Read the model definition and answer for the solid it produces. Units are mm, in the model's axes. A direction names the side the tool comes from. Coordinates: 2 decimals unless noted, no trailing zeros. Loops run counter-clockwise (first coordinate to the right, second up) from the corner with the lowest first, then second, coordinate; pieces in that order, holes last.
from build123d import *

# Parameters (mm, degrees)
F1_DEPTH = 30
F3_D     = 7
F5_D     = 7
F6_W     = 20.071618259
F6_H     = 16.8062914163
F7_DEPTH = 87


with BuildPart() as f1:
    # F0 (on Front) → F1 (new body)
    with BuildSketch(Plane.XZ):
        with BuildLine():
            ThreePointArc((-5.9981474183, 6.1490890598), (-4.2950281931, 1.8104018307), (0, 0))
            Line((0, 0), (40, 0))
            ThreePointArc((40, 0), (44.8583417204, 2.4791313959), (45.7018609438, 7.8678280909))
            Line((45.7018609438, 7.8678280909), (30, 100))
            Line((30, 100), (20, 100))
            Line((20, 100), (10, 100))
            Line((10, 100), (-5.9981474183, 6.1490890598))
        make_face()
        with BuildLine():
            ThreePointArc((30, 100), (20, 111.6119907276), (10, 100))
            Line((10, 100), (20, 100))
            Line((20, 100), (30, 100))
        make_face()
    extrude(amount=F1_DEPTH)

    # F3 (through all)
    with Locations(Plane.XZ.offset(30)):
        with Locations((20, 7.6905470341)):
            Hole(F3_D / 2)

    # F5 (through all)
    with Locations(Plane.XZ.offset(30)):
        with Locations((20, 101.5001014674)):
            Hole(F5_D / 2)

    # F6 (on face) → F7 (cut)
    with BuildSketch(Plane(origin=(0, 0, 0), x_dir=(1, 0, 0), z_dir=(0, 0, -1))):
        with Locations((20.9973212332, 14.0443919227)):
            Rectangle(F6_W, F6_H)
    extrude(amount=-F7_DEPTH, mode=Mode.SUBTRACT)


solid = f1.part
Q1. Which of the six approach directions +Z, -Z, +X, -X, +Y, -Y give full straight-line access (tool end or side, diameter ignored) to faces 5 (the face through (16.66, -26.17, 8.74)), 6 (the face through (21, -22.448, 43))?
Findings below:
face 5: +Y, -Y
face 6: -Z
Q2. A cutting plane is placed at C-C (y = -4.25). Give the vertices of the cut face in (x, z), then the cut area to 3 significant figures.
Findings below:
outline: (-6, 6.15) arc R6 ccw to (0, 0) - (40, 0) arc R6 ccw to (45.7, 7.87) - (30, 100) arc R10.11 ccw (long way) to (10, 100) - close; hole circle Ø7 at (20, 7.69); hole circle Ø7 at (20, 101.5)
area: 3,800 mm2
Q3. Determine the mould class of faces 1 (the face through (10.962, -14, 43)), 2 (the face through (20, 0, 44)), 3 (the face through (-4.342, -14.79, 1.859)), 4 (the face through (37.96, -14.79, 53.29)) for opening direction X: +X half, -X half, draft (parallel to the pull), parting line (faces both ways), or undercut.
Findings below:
face 1: undercut
face 2: draft
face 3: -X half
face 4: +X half
Q4. A cutting plane is placed at A-A (x = 20). Give the vertices of the cut face in (y, z), then the cut area to 3 significant figures.
Findings below:
outline: (-30, 0) - (-22.45, 0) - (-22.45, 4.19) - (-30, 4.19) - close; (-30, 11.19) - (-22.45, 11.19) - (-22.45, 87) - (-5.64, 87) - (-5.64, 11.19) - (0, 11.19) - (0, 98) - (-30, 98) - close; (-30, 105) - (0, 105) - (0, 111.61) - (-30, 111.61) - close; (-5.64, 0) - (0, 0) - (0, 4.19) - (-5.64, 4.19) - close
area: 1,580 mm2
Q5. Flat-ended cylindrical pins translate along their axes: pin 1 Ø3 at (y, z) = (-10, 18.5) entering from -X; pin 2 Ø5 at (y, z) = (-24.5, 14.5) entering from +X; pin 3 Ø1.5 at (x, y) = (23.5, -12) entering from +Z. Find the tip coordinate at first contact, or state that the pin passes through.
Findings below:
pin 1: stops at x = -4.15
pin 2: stops at x = 45
pin 3: stops at z = 111.23
Q6. A cutting plane is placed at D-D (z = 82.5). Give the vertices of the cut face in (x, y).
Findings below:
outline: (7.02, -30) - (32.98, -30) - (32.98, 0) - (7.02, 0) - close; hole (10.96, -22.45) - (31.03, -22.45) - (31.03, -5.64) - (10.96, -5.64) - close
Q7. A cutting plane is placed at B-B (z = 48). Give the vertices of the cut face in (x, y), then the cut area to 3 significant figures.
Findings below:
outline: (1.14, -30) - (38.86, -30) - (38.86, 0) - (1.14, 0) - close; hole (10.96, -22.45) - (31.03, -22.45) - (31.03, -5.64) - (10.96, -5.64) - close
area: 794 mm2
Q8. Straight lines are drawn through the part: probe 1 along Z at (x, y) = (20, -25.5); probe 2 along Y at (x, z) = (25, 83.5); probe 3 along Z at (x, y) = (20, -10.25). For each, find the intervals that lie inside material, in ascending order.
Findings below:
probe 1: z = 0 to 4.19, 11.19 to 98, 105 to 111.61
probe 2: y = -30 to -22.45, -5.64 to 0
probe 3: z = 87 to 98, 105 to 111.61
